Input: part model. Units: mm. Frame: model coordinates. A direction names the side the tool comes from. Give positions to 0.01 mm unless a question says otherwise; leave off trailing zeros. Write each loop counter-clockwise with the first axis right and the second up, starting at its lowest first coordinate (ties: lowest second). Pieces come first, ordered by that corner, then holes. Notation, with made-up numbers: (1, 56.25) -> (33, 56.25) arc R15 ccw to (33, 78.25) -> close; hole circle Ø5 at (12.5, 66.25). An arc over 180 degrees is marked (long way). Return JSON: item names as keys, results as strings. Group by question number.
Item 1: Line query: line 1 (Y direction, x = 0, z = 55); line 2 (Z direction, x = 5, y = 0.75); line 3 (Y direction, x = -0.5, z = 53). Output: solid intervals per line, ascending. Write a range as [from, to].
Item 2: Section B-B, the plane x = 0. Return loops of the section in (y, z).
Item 3: Mould query, pull axis X, two halves, no side actions, for faces 3 (the face through (-3.905, -0.867, 102.535)), 4 (the face through (0, -2, 105)), 5 (the face through (-1.5, 0.07, 53.24)). Classes: released by +X, released by -X, zero draft, split by the parting line, or undercut.
Item 4: Section A-A, the plane y = 0. Return loops of the section in (x, z).
Item 5: Pin query (flat end, axial travel): P1, Ø1, axis at x = 0, z = 94, coming from the -Y side; P2, Ø4, axis at x = 3, z = 44.5, coming from the +Y side; P3, Ø8, axis at x = 5, z = 53.5, coming from the -Y side; P4, Ø1.8, axis at x = 0, y = 0, coming from the +Z side. Return the tip coordinate at first contact, or that it passes through.
Item 6: Section D-D, the plane y = -6.25. Return loops of the section in (x, z).
Item 7: Section C-C, the plane z = 10. Return loops of the section in (x, y).
Item 8: Set-up query: faces 1 (the face through (7, 0, 2)), 2 (the face through (-1.08, -4.88, 51.33)). Return all of +Z, -Z, +X, -X, +Y, -Y with unobstructed straight access to the full face (end or side cutting, diameter ignored); none if empty.
from build123d import *

# Parameters (mm, degrees)
F0_R     = 8.5
F1_DEPTH = 4
F2_R     = 5
F3_DEPTH = 100
F4_W     = 4
F4_H     = 5
F7_DEPTH = 4
F8_R     = 1.5
F9_DEPTH = 114.9


with BuildPart() as f1:
    # F0 (on Top) → F1 (new body)
    with BuildSketch(Plane.XY):
        Circle(F0_R)
    extrude(amount=F1_DEPTH)

    # F2 (on Top) → F3 (join)
    with BuildSketch(Plane.XY):
        Circle(F2_R)
    extrude(amount=F3_DEPTH)

    # F4 (on Right) → F5 (revolve)
    with BuildSketch(Plane.YZ):
        with Locations((2, 102.5)):
            Rectangle(F4_W, F4_H)
    revolve(axis=Axis((0, 0, 102.5), (0, 0, -1)))

    # F6 (on face) → F7 (cut)
    with BuildSketch(Plane(origin=(0, 0, 0), x_dir=(1, 0, 0), z_dir=(0, 0, -1))):
        with BuildLine():
            ThreePointArc((7, -4.821825), (8.5, 0), (7, 4.821825))
            Line((7, 4.821825), (7, -4.821825))
        make_face()
    extrude(amount=-F7_DEPTH, mode=Mode.SUBTRACT)

    # F8 (on face) → F9 (cut)
    with BuildSketch(Plane.XY.offset(105)):
        Circle(F8_R)
    extrude(amount=-F9_DEPTH, mode=Mode.SUBTRACT)


solid = f1.part
Answer below:
{
 "1": {"line 1": "y = [-5, -1.5], [1.5, 5]", "line 2": "z = [0, 4]", "line 3": "y = [-4.97, -1.41], [1.41, 4.97]"},
 "2": {"outline": "(-8.5, 0) -> (-1.5, 0) -> (-1.5, 105) -> (-4, 105) -> (-4, 100) -> (-5, 100) -> (-5, 4) -> (-8.5, 4) -> close; (1.5, 0) -> (8.5, 0) -> (8.5, 4) -> (5, 4) -> (5, 100) -> (4, 100) -> (4, 105) -> (1.5, 105) -> close"},
 "3": {"face 3": "split by the parting line", "face 4": "zero draft", "face 5": "undercut"},
 "4": {"outline": "(-8.5, 0) -> (-1.5, 0) -> (-1.5, 105) -> (-4, 105) -> (-4, 100) -> (-5, 100) -> (-5, 4) -> (-8.5, 4) -> close; (1.5, 0) -> (7, 0) -> (7, 4) -> (5, 4) -> (5, 100) -> (4, 100) -> (4, 105) -> (1.5, 105) -> close"},
 "5": {"P1": "stops at y = -5", "P2": "stops at y = 4.9", "P3": "stops at y = -4.9", "P4": "passes through"},
 "6": {"outline": "(-5.76, 0) -> (5.76, 0) -> (5.76, 4) -> (-5.76, 4) -> close"},
 "7": {"outline": "circle Ø10 at (0, 0); hole circle Ø3 at (0, 0)"},
 "8": {"face 1": "+Z, -Z, +X, +Y, -Y", "face 2": "+Z"}
}
